Input: dimensioned drawing with shaded views. Units: mm. Origin: part minimum x, y, z. A direction names the side the tool comes from. Give positions to 0.01 mm unless a question says otherwise; leave off trailing zeros. Write each loop counter-clockwise with the first axis right and the second up, starting at its lowest first coordinate (ties: lowest second). Pieces come first, ordered by that corner, then holes. Notation, with made-up numbers: (43.25, 12.5) -> (96.25, 12.5) arc R34 cw to (96.25, 45.5) -> close; hole circle Ø8 at (-36.75, 9.5). An arc over 180 degrees is marked (long way). Answer in a Markdown table with one row per item. Add a question column.
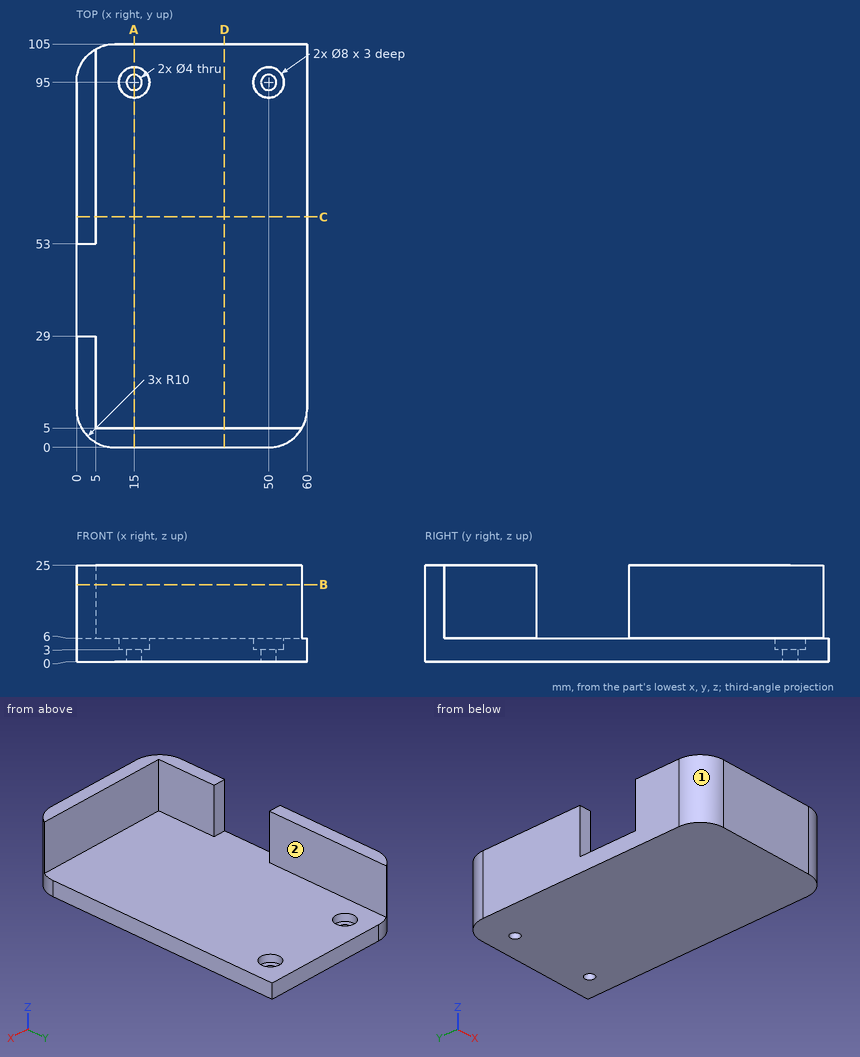
Q1. Section D-D on x = 38.5. Return loops of the section in (y, z).
Q2. Section B-B on z = 20. Return loops of the section in (x, y), and give its area (3 significant figures).
Q3. Line query: probe 1 along X at (y, z) = (95, 4.15); probe 2 along Y at (x, z) = (50, 4.45); probe 3 along X at (y, z) = (61.5, 10.5). Output: solid intervals per line, ascending. Write a range as from..to.
Q4. Section A-A on x = 15. Return loops of the section in (y, z).
Q5. Section C-C on y = 60. Return loops of the section in (x, z), and give its area (3 significant figures).
Q6. Access query for the marked faces 1 and 2. Directions: +Z, -Z, +X, -X, +Y, -Y. A direction counts if a zero-diameter tool reaches every point of the face in a straight line with its end or side. Return the directions, or none.
Q7. Contact query for flat-ended pins moving along their axis: pin 1 Ø5 at (y, z) = (52.5, 13) entering from +X; pin 2 Ø18 at (x, y) = (25.5, 48.5) entering from +Z; pin 3 Ø7 at (x, y) = (15, 95) entering from +Z. Output: stop coordinate, or through.
Checks:
| question | item | result |
|---|---|---|
| 1 | outline | (0, 0) -> (105, 0) -> (105, 6) -> (5, 6) -> (5, 25) -> (0, 25) -> close |
| 2 | outline | (0, 10) arc R10 ccw to (10, 0) -> (50, 0) arc R10 ccw to (58.66, 5) -> (5, 5) -> (5, 29) -> (0, 29) -> close; (0, 53) -> (5, 53) -> (5, 103.66) arc R10 ccw to (0, 95) -> close |
| 2 | area | 620 mm^2 |
| 3 | probe 1 | 0..11, 19..46, 54..60 |
| 3 | probe 2 | 0..91, 99..105 |
| 3 | probe 3 | 0..5 |
| 4 | outline | (0, 0) -> (93, 0) -> (93, 3) -> (91, 3) -> (91, 6) -> (5, 6) -> (5, 25) -> (0, 25) -> close; (97, 0) -> (105, 0) -> (105, 6) -> (99, 6) -> (99, 3) -> (97, 3) -> close |
| 5 | outline | (0, 0) -> (60, 0) -> (60, 6) -> (5, 6) -> (5, 25) -> (0, 25) -> close |
| 5 | area | 455 mm^2 |
| 6 | face 1 | +Z, -Z, -X, -Y |
| 6 | face 2 | +Z, +X, +Y |
| 7 | pin 1 | x = 5 |
| 7 | pin 2 | z = 6 |
| 7 | pin 3 | z = 3 |
